Part model, mm, in its own coordinate system. A direction names the side the tool comes from. Round coordinates to 2 decimals unless told otherwise and drop trailing zeros. Loops run counter-clockwise (first coordinate to the right, second up) from the corner with the lowest first, then second, coordinate; pieces in that order, holes last.
1) Band-saw the part on A-A, the plane y = 192. Write the cut outline in (x, z).
2) Band-saw the part on B-B, the plane y = 284.5. Write the cut outline in (x, z), then the cut area to 3 significant figures.
3) Mould opens along Z. For faces 1 (the flat face through (94, 300, 15)), 2 (the cylindrical face through (22.4, 211.83, -24.65)), 3 (the flat face through (94, -87, 51.62)) say: +Z half, -Z half, draft (parallel to the pull), parting line (faces both ways), or undercut.
4) Band-saw the part on C-C, the plane z = -28.5. Write the cut outline in (x, y).
5) Band-saw the part on D-D, the plane x = 175. State how many separate pieces and enclosed holes the cut face has, then the cut area to 3 significant figures.
6) Probe line 1 (Y direction, x = 15, z = 10); line 2 (X direction, y = 99, z = 7); line 3 (Z direction, x = 83, y = 271). List the from-to ranges inside material, lowest first.
7) Drop flat-ended pins along their axis: P1, Ø22.5, axis at x = 60, z = 43, coming from the +Y side; P2, Ø4, axis at x = 77.5, y = 153.5, coming from the +Z side; P3, Ø13, axis at x = 175, y = 99.5, coming from the -Z side. Give the stop position or say it passes through.
8) 3-axis set-ups, long thin cutter, end or side, ignore diameter. For faces 4 (the cylindrical face through (179.74, 205.52, -24.65)), 5 (the flat face through (94, -177.45, 26)), 6 (the flat face through (94, 0, 41)): which of +Z, -Z, +X, -X, +Y, -Y reach the whole face in a straight line?
from build123d import *

# Parameters (mm, degrees)
ESQUISSE1_W             = 190
ESQUISSE1_H             = 300
BOSS_EXTRU_1_DEPTH      = 31
ESQUISSE2_R             = 5
ENL_V_MAT_EXTRU_1_DEPTH = 357.456168413
ESQUISSE3_W             = 190
ESQUISSE3_H             = 51.62
BOSS_EXTRU_2_DEPTH      = 177.45
ESQUISSE4_R             = 20
BOSS_EXTRU_3_DEPTH      = 50
ESQUISSE6_R             = 20
R_VOLUTION1_ANGLE       = 180


with BuildPart() as part:
    # Esquisse1 → Boss.-Extru.1 (new body)
    with BuildSketch(Plane.XY):
        with Locations((95, 150)):
            Rectangle(ESQUISSE1_W, ESQUISSE1_H)
    extrude(amount=BOSS_EXTRU_1_DEPTH)

    # Esquisse2 → Enlèv. mat.-Extru.1 (cut, through all)
    with BuildSketch(Plane(origin=(0, 0, 0), x_dir=(-1, 0, 0), z_dir=(0, 0, -1))):
        with Locations((-175, 284.5)):
            Circle(ESQUISSE2_R)
        with Locations((-15, 284.5)):
            Circle(ESQUISSE2_R)
        with Locations((-175, 99.5)):
            Circle(ESQUISSE2_R)
        with Locations((-15, 99.5)):
            Circle(ESQUISSE2_R)
    extrude(amount=-ENL_V_MAT_EXTRU_1_DEPTH, mode=Mode.SUBTRACT)

    # Esquisse3 → Boss.-Extru.2 (add)
    with BuildSketch(Plane.XZ):
        with Locations((95, 25.81)):
            Rectangle(ESQUISSE3_W, ESQUISSE3_H)
    extrude(amount=BOSS_EXTRU_2_DEPTH)

    # Esquisse4 → Boss.-Extru.3 (add)
    with BuildSketch(Plane(origin=(0, 0, 0), x_dir=(-1, 0, 0), z_dir=(0, 0, -1))):
        with Locations((-165, 192)):
            Circle(ESQUISSE4_R)
    boss_extru_3 = extrude(amount=BOSS_EXTRU_3_DEPTH)

    # Symétrie1: Boss.-Extru.3 across plane
    add(boss_extru_3.mirror(Plane(origin=(95, 0, 0), x_dir=(0, 0, 1), z_dir=(1, 0, 0))))

    # Esquisse6 → Révolution1 (revolve)
    with BuildSketch(Plane(origin=(0, 0, -50), x_dir=(-1, 0, 0), z_dir=(0, 0, -1))):
        with Locations(Location((-165, 192, 0), (0, 0, 180))):
            Circle(ESQUISSE6_R)
    revolve(axis=Axis((95, -201.3225, -50), (0, 1, 0)), revolution_arc=R_VOLUTION1_ANGLE)


solid = part.part
Reported:
1. outline: (0, 0) - (5, 0) - (5, -50) arc R90 ccw to (185, -50) - (185, 0) - (190, 0) - (190, 31) - (0, 31) - close; hole (45, -50) arc R50 ccw to (145, -50) - (145, 0) - (45, 0) - close
2. outline: (0, 0) - (10, 0) - (10, 31) - (0, 31) - close; (20, 0) - (170, 0) - (170, 31) - (20, 31) - close; (180, 0) - (190, 0) - (190, 31) - (180, 31) - close
2. area: 5,270 mm2
3. face 1: draft
3. face 2: undercut
3. face 3: +Z half
4. outline: circle Ø40 at (25, 192); circle Ø40 at (165, 192)
5. separate pieces: 3
5. enclosed holes: 0
5. area: 20,700 mm2
6. line 1: y = -177.45 to 94.5, 104.5 to 279.5, 289.5 to 300
6. line 2: x = 0 to 10.03, 19.97 to 170.03, 179.97 to 190
6. line 3: z = 0 to 31
7. P1: stops at y = 0
7. P2: stops at z = 31
7. P3: stops at z = 0
8. face 4: none
8. face 5: +Z, -Z, +X, -X, -Y
8. face 6: +Z, +X, -X, +Y
